Input: part model. Units: mm. Frame: model coordinates. Face numbers are marked on the shaded views. A direction names the side the tool comes from. Coordinates: 2 decimals unless noted, no trailing zeros. Write each loop counter-clockwise with the first axis right and the second up, starting at its lowest first coordinate (ties: lowest second). Pieces come first, ordered by that corner, then holes. Notation, with made-up numbers: M 85.25,38 L 116.25,38 A19 ccw 116.25,56 Z; hole C 71.25,56 d8. An arc over 180 degrees is marked long. Use one line per item in the form item = value.
from build123d import *

# Parameters (mm, degrees)
F0_W     = 1219.2
F0_H     = 558.8
F1_DEPTH = 12.7
F3_DEPTH = 3.175


# Not quite as in the source:
# - ends of sketch curves that miss each other by under 0.0002 mm in the source are joined


with BuildPart() as f1:
    # F0 (on Front) → F1 (new body)
    with BuildSketch(Plane.XZ):
        Rectangle(F0_W, F0_H)
    extrude(amount=F1_DEPTH)

    # F2 (on face) → F3 (cut)
    with BuildSketch(Plane.XZ.offset(12.7)):
        Polygon((-110.776385, 136.9130104), (-147.738846, 136.9130104), (-147.738846, 66.8081214), (-85.6601792, -32.312991), (-9.521317, -115.3251186), (-9.521317, -158.7848488), (9.521317, -158.7848488), (9.521317, -115.3251186), (85.6601538, -32.312991), (147.738846, 66.8081214), (147.738846, 136.9130104), (110.7763596, 136.9130104), (9.470136, -102.9111988), (8.4179664, -24.1473228), (68.9105556, 59.2761832), (107.1551832, 136.9130104), (2.6089356, 136.9130104), (2.900426, 89.6063994), (24.4521482, 19.6980556), (-0.0642366, -18.3666638), (-24.4521482, 19.6980556), (-3.439668, 89.6063994), (-3.0142434, 136.9130104), (-107.1551832, 136.9130104), (-68.9105556, 59.2761832), (-8.4179918, -24.1473228), (-9.470136, -102.9111988), align=None)
        Polygon((-28.2203906, -158.7848488), (-147.738846, 59.252739), (-147.738846, -158.7848488), align=None)
        Polygon((147.738846, -158.7848488), (147.738846, 59.252739), (28.2203652, -158.7848488), align=None)
        with BuildLine():
            ThreePointArc((-109.8671422064, -179.8267368126), (-95.356903919, -186.4744799885), (-89.4000786424, -201.2817666107))
            Line((-89.4000786424, -201.2817666107), (-86.0775266, -201.2817666))
            Line((-86.0775266, -201.2817666), (-87.228807, -174.6107506))
            Line((-87.228807, -174.6107506), (-90.1839446, -174.6107506))
            Line((-90.1839446, -174.6107506), (-93.0793668, -180.8493462))
            ThreePointArc((-93.0793668, -180.8493462), (-102.7053794925, -175.5791240788), (-113.6444505241, -174.7004700875))
            ThreePointArc((-113.6444505241, -174.7004700875), (-140.7442467729, -209.1274434593), (-113.39827807, -243.3592184707))
            ThreePointArc((-113.39827807, -243.3592184707), (-93.1382802166, -237.533313942), (-84.4416180716, -218.3297640292))
            Line((-84.4416180716, -218.3297640292), (-87.6078766, -218.329764))
            ThreePointArc((-87.6078766, -218.329764), (-93.9825550775, -232.5723606205), (-108.5038975848, -238.2836063253))
            ThreePointArc((-108.5038975848, -238.2836063253), (-122.8229554836, -232.9071157052), (-128.4500788749, -218.68467849))
            Line((-128.4500788749, -218.68467849), (-128.450086, -203.0753622))
            ThreePointArc((-128.450086, -203.0753622), (-124.1111022303, -187.4924501184), (-109.8671422064, -179.8267368126))
        make_face()
        with BuildLine():
            Line((-55.665624, -238.077629), (-55.665624, -241.4936496))
            Line((-55.665624, -241.4936496), (-25.422352, -241.4936496))
            Line((-25.422352, -241.4936496), (-25.422352, -238.077629))
            Line((-25.422352, -238.077629), (-32.919924, -238.077629))
            ThreePointArc((-32.919924, -238.077629), (-35.0246805086, -237.2058103086), (-35.8964992, -235.1010538))
            Line((-35.8964992, -235.1010538), (-35.8964738, -182.243603))
            ThreePointArc((-35.8964738, -182.243603), (-35.0246805086, -180.1388464914), (-32.919924, -179.2670278))
            Line((-32.919924, -179.2670278), (-25.422352, -179.2670532))
            Line((-25.422352, -179.2670532), (-25.422352, -175.8510072))
            Line((-25.422352, -175.8510072), (-55.665624, -175.8510072))
            Line((-55.665624, -175.8510072), (-55.665624, -179.2670532))
            Line((-55.665624, -179.2670532), (-48.0573588, -179.2670532))
            ThreePointArc((-48.0573588, -179.2670532), (-45.9526022914, -180.1388464914), (-45.0807836, -182.243603))
            Line((-45.0807836, -182.243603), (-45.080809, -235.1010538))
            ThreePointArc((-45.080809, -235.1010538), (-45.9526022914, -237.2058103086), (-48.0573588, -238.077629))
            Line((-48.0573588, -238.077629), (-55.665624, -238.077629))
        make_face()
        with BuildLine():
            Line((31.9159128, -205.8210006), (23.7701836, -205.8210006))
            Line((23.7701836, -205.8210006), (23.7701836, -182.2325286))
            ThreePointArc((23.7701836, -182.2325286), (24.6423974564, -180.1274129149), (26.7478255999, -179.2559789912))
            Line((26.7478255999, -179.2559789912), (41.0262324, -179.2611096))
            ThreePointArc((41.0262324, -179.2611096), (51.1481998687, -186.6406443843), (55.0079383919, -198.557616598))
            Line((55.0079383919, -198.557616598), (58.1934574, -198.5576166))
            Line((58.1934574, -198.5576166), (57.3842134, -175.8510072))
            Line((57.3842134, -175.8510072), (5.1603656, -175.8321858))
            Line((5.1603656, -175.8321858), (5.153533, -179.2482064))
            Line((5.153533, -179.2482064), (11.6103908, -179.2505178))
            ThreePointArc((11.6103908, -179.2505178), (13.7144412242, -180.1227226778), (14.5858738, -182.227093))
            Line((14.5858738, -182.227093), (14.5858738, -235.1010538))
            ThreePointArc((14.5858738, -235.1010538), (13.7140551086, -237.2058103086), (11.6092986, -238.077629))
            Line((11.6092986, -238.077629), (3.801745, -238.077629))
            Line((3.801745, -238.077629), (3.801745, -241.4936496))
            Line((3.801745, -241.4936496), (35.4731574, -241.4936496))
            Line((35.4731574, -241.4936496), (35.4731574, -238.077629))
            Line((35.4731574, -238.077629), (26.7467588, -238.077629))
            ThreePointArc((26.7467588, -238.077629), (24.6420022914, -237.2058103086), (23.7701836, -235.1010538))
            Line((23.7701836, -235.1010538), (23.7701836, -209.2370212))
            Line((23.7701836, -209.2370212), (31.9159128, -209.2370212))
            ThreePointArc((31.9159128, -209.2370212), (37.6830347812, -213.8514597759), (39.8617861947, -220.9087784101))
            Line((39.8617861947, -220.9087784101), (39.8617948, -222.7084954))
            Line((39.8617948, -222.7084954), (43.1732436, -222.7084954))
            Line((43.1732436, -222.7084954), (43.1732436, -193.1940002))
            Line((43.1732436, -193.1940002), (39.8617948, -193.1940002))
            Line((39.8617948, -193.1940002), (39.8617948, -194.1492434))
            ThreePointArc((39.8617948, -194.1492434), (37.6830347812, -201.2065620241), (31.9159128, -205.8210006))
        make_face()
        with BuildLine():
            Line((106.7346608, -182.243603), (106.7346608, -235.1010538))
            ThreePointArc((106.7346608, -235.1010538), (105.8628421086, -237.2058103086), (103.7580856, -238.077629))
            Line((103.7580856, -238.077629), (96.1487536, -238.077629))
            Line((96.1487536, -238.077629), (96.1487536, -241.4936496))
            Line((96.1487536, -241.4936496), (126.6514358, -241.4936496))
            Line((126.6514358, -241.4936496), (126.6514358, -238.077629))
            Line((126.6514358, -238.077629), (118.8955458, -238.077629))
            ThreePointArc((118.8955458, -238.077629), (116.7907892914, -237.2058103086), (115.9189706, -235.1010538))
            Line((115.9189706, -235.1010538), (115.9189706, -182.243603))
            ThreePointArc((115.9189706, -182.243603), (116.7907892914, -180.1388464914), (118.8955458, -179.2670278))
            Line((118.8955458, -179.2670278), (124.14758, -179.2670532))
            ThreePointArc((124.14758, -179.2670532), (132.9675370035, -188.3940946035), (135.9963466509, -200.7197153285))
            Line((135.9963466509, -200.7197153285), (139.3194572, -200.7197154))
            Line((139.3194572, -200.7197154), (137.8614718, -175.8510072))
            Line((137.8614718, -175.8510072), (84.7921596, -175.8510072))
            Line((84.7921596, -175.8510072), (83.3341742, -200.7197154))
            Line((83.3341742, -200.7197154), (86.6572816, -200.7197154))
            ThreePointArc((86.6572816, -200.7197154), (89.6860943965, -188.3940946035), (98.5060445889, -179.2670418075))
            Line((98.5060445889, -179.2670418075), (103.7580856, -179.2670532))
            ThreePointArc((103.7580856, -179.2670532), (105.8628421086, -180.1388464914), (106.7346608, -182.243603))
        make_face()
        Polygon((-2.0544028, 243.6519638), (-2.9994959967, 138.552993536), (2.5988306881, 138.552993536), (1.9512534, 243.6519638), align=None)
        Polygon((-164.3414798, 89.5408928), (-148.8750427961, 61.3255006909), (-148.8750427961, 68.7675664065), (-161.7813884, 91.0253958), align=None)
        Polygon((-111.3482406, 146.2952116), (-114.2778258, 145.2020718), (-111.0982667862, 137.6750104), (-107.4957333194, 137.6750104), align=None)
        Polygon((111.0982437212, 137.6750104), (114.2778258, 145.2020718), (111.3482406, 146.2952116), (107.4957333194, 137.6750104), align=None)
        Polygon((164.3414798, 89.5408928), (161.7813884, 91.0253958), (148.5202014446, 68.1556195002), (148.5202014446, 60.6781642768), align=None)
    extrude(amount=-F3_DEPTH, mode=Mode.SUBTRACT)


solid = f1.part
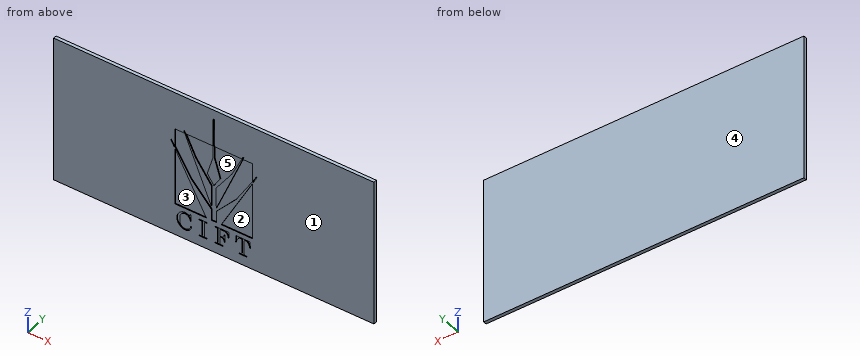
(1) Section query B-B on z = -58. Return the cut outline in (x, y) (3 decimals).
Computed:
outline = M -609.6,-12.7 L -147.739,-12.7 L -147.739,-9.525 L -83.466,-9.525 L -83.466,-12.7 L -62.1,-12.7 L -62.1,-9.525 L -28.441,-9.525 L -28.441,-12.7 L -8.87,-12.7 L -8.87,-9.525 L 8.87,-9.525 L 8.87,-12.7 L 28.441,-12.7 L 28.441,-9.525 L 62.1,-9.525 L 62.1,-12.7 L 83.466,-12.7 L 83.466,-9.525 L 147.739,-9.525 L 147.739,-12.7 L 609.6,-12.7 L 609.6,0 L -609.6,0 Z
(2) Section query A-A on z = 5. Return the cut outline in (x, y) (3 decimals).
Computed:
outline = M -609.6,-12.7 L -147.739,-12.7 L -147.739,-9.525 L -118,-9.525 L -118,-12.7 L -109.029,-12.7 L -109.029,-9.525 L -55.054,-9.525 L -55.054,-12.7 L -29.553,-12.7 L -29.553,-9.525 L -15.035,-9.525 L -15.035,-12.7 L 14.986,-12.7 L 14.986,-9.525 L 29.553,-9.525 L 29.553,-12.7 L 55.054,-12.7 L 55.054,-9.525 L 109.029,-9.525 L 109.029,-12.7 L 118,-12.7 L 118,-9.525 L 147.739,-9.525 L 147.739,-12.7 L 609.6,-12.7 L 609.6,0 L -609.6,0 Z
(3) Pull-direction query (Z, two-part tool) for the marked faces 1, 2 and 3; classes: pulls with the +Z half, pulls with the -Z half, needs draft (parallel to the pull), parting line crosses it, or undercut.
Computed:
face_1 = needs draft
face_2 = undercut
face_3 = undercut
(4) Line query: probe 1 along X at (y, z) = (-11.25, 163); probe 2 along Y at (x, z) = (-89.5, 50) (3 decimals). Output: solid intervals per line, ascending.
Computed:
probe_1 = -609.6 to -2.78, 2.45 to 609.6
probe_2 = -9.525 to 0
(5) Set-up query: the marked faces 4 and 5. Return all of +Z, -Z, +X, -X, +Y, -Y with unobstructed straight access to the full face (end or side cutting, diameter ignored); none if empty.
Computed:
face_4 = +Z, -Z, +X, -X, +Y
face_5 = -Y
